Autodesk Fusion 360 part; units mm, degrees
sketch "Sketch1" plane through (0, 0, 0) normal (1, 0, 0) x (0, 1, 0)
  line L0 (0, 0) -> (0, 40)
  line L1 (0, 40) -> (20, 20)
  line L2 (38.614, 36.3802) -> (38.614, 30)
  line L3 (20, 20) -> (20, 0)
  line L4 (20, 0) -> (20, -50)
  line L5 (20, -50) -> (60, -50)
  line L6 (60, -50) -> (60, -70)
  line L7 (60, -70) -> (0, -70)
  line L8 (0, -70) -> (0, 40)
revolve "Revolve1" add sketch "Sketch1" angle 360 about axis through (0, 0, 1.75) along (0, 0, 1)
sketch "Sketch2" plane through (0, 0, 0) normal (1, 0, 0) x (0, 1, 0)
  line L0 (60, -50) -> (40, -50)
  line L1 (40, -50) -> (40, -70)
  line L2 (40, -70) -> (60, -70)
  line L3 (60, -70) -> (60, -50)
revolve "Revolve2" cut sketch "Sketch2" angle 360 about axis through (0, 60, -70) along (0, 0, 1)
mirror "Mirror1" about plane through (0, 0, 0) normal (0, 1, 0) of "Revolve2"
The listing builds one solid part. Answer for the finished solid, in the listing's coordinates (mm). A direction names the side the tool comes from. Give positions to 0.01 mm unless a question says otherwise; leave off trailing zeros. Write each loop counter-clockwise with the first axis right and the second up, starting at its lowest first coordinate (ties: lowest second). Pieces come first, ordered by that corner, then holes. Notation, with made-up numbers: (25, -9) -> (57, -9) arc R20 cw to (57, 25) -> close; hole circle Ø2 at (-25.5, 16.5). An arc over 180 degrees is marked (long way). One line per question, with ' | ' between items. Start each with the question number.
1. For a pull along X with two mould halves and no side action, classify faces 1 (the cylindrical face through (0, -40, -60)), 2 (the cylindrical face through (-59.99, -1.04, -60.14)), 3 (the cylindrical face through (59.99, 1.04, -60.14)), 4 (the conical face through (-5.56, -1.235, 34.304)) as pulls with the +X half, pulls with the -X half, needs draft (parallel to the pull), parting line crosses it, or undercut.
2. For faces 5 (the cylindrical face through (-19.524, -4.336, -15.49)), 6 (the flat face through (-1, -1, -70)), determine the directions among +Z, -Z, +X, -X, +Y, -Y from which every point of the face is accessible in a straight line to the end or side of a thin tool.
3. Section A-A (z = 18) is taken. Determine the outline of the cut face in (x, y), plus the area to 3 significant figures.
4. Find the intervals of material crossed by probe 1 along Z at (x, y) = (-47, -10.5); probe 2 along Z at (x, y) = (13, -5.5); probe 3 along X at (y, z) = (-8, -61.5), in increasing order.
5. Given pin 1 Ø5 at (y, z) = (15, -24) entering from -X; pin 2 Ø5 at (x, z) = (-15, -37.5) entering from +Y; pin 3 Ø5 at (x, z) = (-21, -27) entering from +Y, each flat-ended and moving along its own axis, determine where each tip first touches the part or whether it passes through.
Response values:
1) face 1: undercut | face 2: pulls with the -X half | face 3: pulls with the +X half | face 4: parting line crosses it
2) face 5: +Z | face 6: -Z, +X, -X, +Y, -Y
3) outline: circle Ø40 at (0, 0) | area: 1,260 mm2
4) probe 1: -70 to -50 | probe 2: -70 to 25.88 | probe 3: -59.46 to 59.46
5) pin 1: x = -15.61 | pin 2: y = 15.61 | pin 3: y = 7.6
